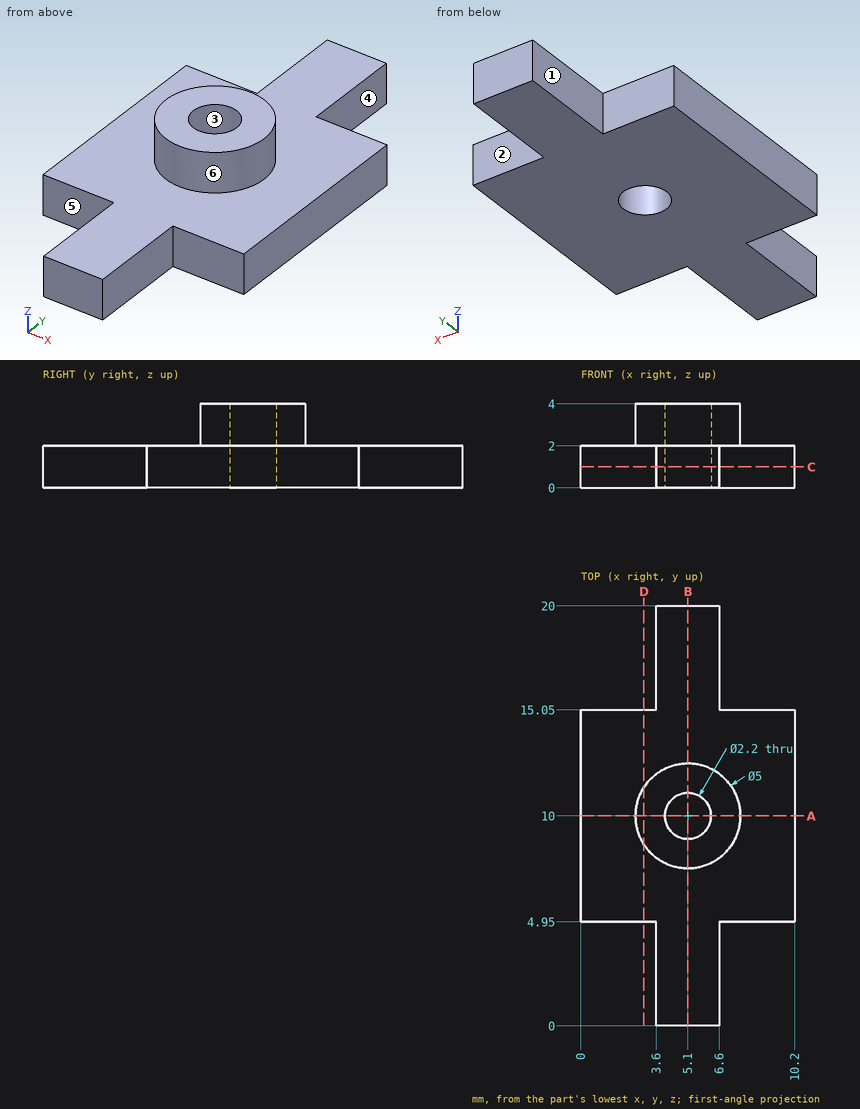
For this review, use the dimensioned drawing (mm, ordinates from the lowest corner) and the shaded views. A direction names the side the tool comes from. Round coordinates to 2 decimals unless told otherwise and drop trailing zeros. Write each loop counter-clockwise with the first axis right and the second up, starting at its lowest first coordinate (ties: lowest second). Pieces come first, ordered by that corner, then holes. Notation, with made-up numbers: (11.5, 28.25) - (19.5, 28.25) arc R31 ccw to (19.5, 66.25) - close; hole circle Ø4 at (-37, 54). An arc over 180 degrees is marked (long way). Use CSV: the item, a comma, the result in double quotes.
1) The part is to be moulded in two halves that separate along X. For the marked faces 1, 2 and 3, say which applies: pulls with the +X half, pulls with the -X half, needs draft (parallel to the pull), parting line crosses it, or undercut.
Conclusion:
face 1,"pulls with the -X half"
face 2,"needs draft"
face 3,"undercut"
2) Add section D-D on x = 3. Write out the cut boundary in (y, z), and give its area (3 significant figures).
Conclusion:
outline,"(4.95, 0) - (15.05, 0) - (15.05, 2) - (11.36, 2) - (11.36, 4) - (8.64, 4) - (8.64, 2) - (4.95, 2) - close"
area,"25.6 mm^2"
3) For the marked faces 4, 5 and 6, list the 3-axis set-ups (+Z, -Z, +X, -X, +Y, -Y) from which the entire face can be reached by the end or side of a thin tool; tool diameter is ignored.
Conclusion:
face 4,"+Z, -Z, +X, +Y"
face 5,"+Z, -Z, -X, -Y"
face 6,"+Z"
4) Add section C-C on z = 1. Write out the cut boundary in (x, y).
Conclusion:
outline,"(0, 4.95) - (3.6, 4.95) - (3.6, 0) - (6.6, 0) - (6.6, 4.95) - (10.2, 4.95) - (10.2, 15.05) - (6.6, 15.05) - (6.6, 20) - (3.6, 20) - (3.6, 15.05) - (0, 15.05) - close; hole circle Ø2.2 at (5.1, 10)"
5) Add section A-A on y = 10. Write out the cut boundary in (x, z), and give its area (3 significant figures).
Conclusion:
outline,"(0, 0) - (4, 0) - (4, 4) - (2.6, 4) - (2.6, 2) - (0, 2) - close; (6.2, 0) - (10.2, 0) - (10.2, 2) - (7.6, 2) - (7.6, 4) - (6.2, 4) - close"
area,"21.6 mm^2"
6) Add section B-B on x = 5.1. Write out the cut boundary in (y, z), and give its area (3 significant figures).
Conclusion:
outline,"(0, 0) - (8.9, 0) - (8.9, 4) - (7.5, 4) - (7.5, 2) - (0, 2) - close; (11.1, 0) - (20, 0) - (20, 2) - (12.5, 2) - (12.5, 4) - (11.1, 4) - close"
area,"41.2 mm^2"
7) Clearance check with flat-ended pins moving along their axes: pin 1 Ø2 at (y, z) = (17.5, 0.5) entering from -X; pin 2 Ø1.6 at (y, z) = (1.5, 1) entering from +X; pin 3 Ø2 at (x, z) = (2, 1.5) entering from +Y. State where each tip first meets the part, or that it passes through.
Conclusion:
pin 1,"stops at x = 3.6"
pin 2,"stops at x = 6.6"
pin 3,"stops at y = 15.05"
8) Wall thickness on line 1 along X through (y, z) = (10, 2.1); line 2 along Y through (x, z) = (5, 1.8); line 3 along X through (y, z) = (10, 1): over which ranges is each line inside the solid? List them lowest first. Write a range as from..to.
Conclusion:
line 1,"x = 2.6..4, 6.2..7.6"
line 2,"y = 0..8.9, 11.1..20"
line 3,"x = 0..4, 6.2..10.2"
